```python
from build123d import *

# Parameters (mm, degrees)
SKETCH1_R           = 12.0269
BOSS_EXTRUDE1_DEPTH = 23.3172
SKETCH3_W           = 3.175
SKETCH3_H           = 19.05
BOSS_EXTRUDE3_DEPTH = 23.9903
CUT_EXTRUDE1_DEPTH  = 10


with BuildPart() as part:
    # Sketch1 → Boss-Extrude1 (new, symmetric)
    with BuildSketch(Plane(origin=(0, 0, 0), x_dir=(1, 0, 0), z_dir=(0, 1, 0))):
        with Locations(Location((0, 0, 0), (0, 0, 90))):
            Circle(SKETCH1_R)
    extrude(amount=BOSS_EXTRUDE1_DEPTH, both=True)

    # Sketch3 → Boss-Extrude3 (add)
    with BuildSketch(Plane(origin=(0, 23.3172, 0), x_dir=(1, 0, 0), z_dir=(0, 1, 0))):
        Rectangle(SKETCH3_W, SKETCH3_H)
    boss_extrude3 = extrude(amount=BOSS_EXTRUDE3_DEPTH)

    # Sketch4 → Cut-Extrude1 (cut)
    with BuildSketch(Plane(origin=(1.5875, 0, 0), x_dir=(0, 0, -1), z_dir=(1, 0, 0))):
        with BuildLine():
            Line((4.4704, 36.2331), (4.4704, 35.6489))
            ThreePointArc((4.4704, 35.6489), (0, 31.1785), (-4.4704, 35.6489))
            Line((-4.4704, 35.6489), (-4.4704, 36.2331))
            ThreePointArc((-4.4704, 36.2331), (0, 40.7035), (4.4704, 36.2331))
        make_face()
        with BuildLine():
            Line((4.4704, -36.2331), (4.4704, -35.6489))
            ThreePointArc((4.4704, -35.6489), (0, -31.1785), (-4.4704, -35.6489))
            Line((-4.4704, -35.6489), (-4.4704, -36.2331))
            ThreePointArc((-4.4704, -36.2331), (0, -40.7035), (4.4704, -36.2331))
        make_face()
    cut_extrude1 = extrude(amount=-CUT_EXTRUDE1_DEPTH, mode=Mode.SUBTRACT)

    # Mirror1: Boss-Extrude3, Cut-Extrude1 across plane
    add(boss_extrude3.mirror(Plane.ZX))
    add(cut_extrude1.mirror(Plane.ZX), mode=Mode.SUBTRACT)


solid = part.part
```
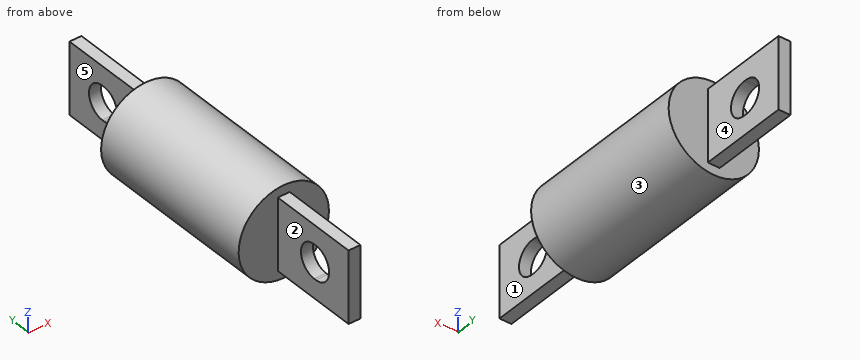
Source: CAD feature listing. Evaluate the final solid. Frame: model axes, mm. Face numbers are marked on the shaded views. A direction names the side the tool comes from. Round coordinates to 2 decimals unless told otherwise and drop trailing zeros. Order: outer loops, then holes, each group sorted by start corner. A loop starts at its lowest first (then second) coordinate and runs counter-clockwise, first axis right, second up. Notation, with made-up numbers: (44, -18) -> (58, -18) arc R23 cw to (58, -5) -> close; hole circle Ø4 at (-35, 4). An arc over 180 degrees is marked (long way). One line per item, written item: value. Start each with the question number.
Q1. Pin query (flat end, axial travel): pin 1 (5.5 mm diameter, centred on y = -39.5, z = -3.5, fed in from +X); pin 2 (1.6 mm diameter, centred on x = 0, y = 29.5, fed in from -Z) (3 decimals); pin 3 (1 mm diameter, centred on x = 0.5, y = -38.5, fed in from +Z) (3 decimals); pin 4 (1 mm diameter, centred on x = 3, y = 29.5, fed in from +Z). Return the tip coordinate at first contact, or that it passes through.
Q2. Section query D-D (x = 7). Return the cut outline in (y, z), plus the area to 3 significant figures.
Q3. Material intervals for probe 1 along Y at (x, z) = (-3, 9); probe 2 along X at (y, z) = (-42.5, -5.5); probe 3 along Z at (x, y) = (1.5, 25) (3 decimals), sorted ascending.
Q4. Section query C-C (y = 11). Return the cut outline in (x, z), plus the area to 3 significant figures.
Q5. Access query for the marked faces 1, 2, 3, 4 and 5. Directions: +Z, -Z, +X, -X, +Y, -Y. A direction counts if a zero-diameter tool reaches every point of the face in a straight line with its end or side. Return the directions, or none.
Q6. Section query B-B (x = 0). Return the cut outline in (y, z) (1 decimal).
Q7. Section query A-A (z = 0). Return the cut outline in (x, y).
Findings below:
1. pin 1: x = 1.59
1. pin 2: z = -9.525
1. pin 3: z = 9.525
1. pin 4: through
2. outline: (-23.32, -9.78) -> (23.32, -9.78) -> (23.32, 9.78) -> (-23.32, 9.78) -> close
2. area: 912 mm²
3. probe 1: -23.32 to 23.32
3. probe 2: -1.59 to 1.59
3. probe 3: -9.525 to 9.525
4. outline: circle Ø24.05 at (0, 0)
4. area: 454 mm²
5. face 1: +Z, -Z, +X, -Y
5. face 2: +Z, -Z, -X, -Y
5. face 3: +Y, -Y
5. face 4: +Z, -Z, +X, +Y
5. face 5: +Z, -Z, -X, +Y
6. outline: (-47.3, -9.5) -> (-23.3, -9.5) -> (-23.3, -12) -> (23.3, -12) -> (23.3, -9.5) -> (47.3, -9.5) -> (47.3, 9.5) -> (23.3, 9.5) -> (23.3, 12) -> (-23.3, 12) -> (-23.3, 9.5) -> (-47.3, 9.5) -> close; hole (-36.2, -4.5) -> (-35.6, -4.5) arc R4.5 ccw to (-35.6, 4.5) -> (-36.2, 4.5) arc R4.5 ccw to start; hole (35.6, -4.5) -> (36.2, -4.5) arc R4.5 ccw to (36.2, 4.5) -> (35.6, 4.5) arc R4.5 ccw to start
7. outline: (-12.03, -23.32) -> (-1.59, -23.32) -> (-1.59, -31.18) -> (1.59, -31.18) -> (1.59, -23.32) -> (12.03, -23.32) -> (12.03, 23.32) -> (1.59, 23.32) -> (1.59, 31.18) -> (-1.59, 31.18) -> (-1.59, 23.32) -> (-12.03, 23.32) -> close; (-1.59, -47.31) -> (1.59, -47.31) -> (1.59, -40.7) -> (-1.59, -40.7) -> close; (-1.59, 40.7) -> (1.59, 40.7) -> (1.59, 47.31) -> (-1.59, 47.31) -> close
